Design review of the part built by this model. Coordinates are the model's own, in mm. A direction names the side the tool comes from. Give positions to 0.01 mm unless a question says otherwise; leave off trailing zeros. Loops run counter-clockwise (first coordinate to the right, second up) from the corner with the lowest first, then second, coordinate; pieces in that order, holes last. Notation, with made-up numbers: M 25,-34 L 83,-34 A19 cw 83,-18 Z; hole C 34,-33.75 d4. An arc over 180 degrees is marked long. Use a Markdown table: item, result. Add a question column.
(1) Insertion check: pin 1 Ø2 at (y, z) = (4, 2) entering from +X; pin 2 Ø0.6 at (x, z) = (1, 2.5) entering from -Y; pin 3 Ø2 at (y, z) = (3, 4.5) entering from -X. Each pin has a flat end and moves straight along its axis. Give the tip position at first contact, or say it passes through.
(2) Draft analysis for pull direction X (two halves, no side actions). For faces 3 (the face through (3, 56, 3)), 4 (the face through (1.5, 3, 4)), 5 (the face through (2.766, 33.785, 3.549)), state which applies: pulls with the +X half, pulls with the -X half, needs draft (parallel to the pull), parting line crosses it, or undercut.
(3) For probe 1 along Y at (x, z) = (3, 5); probe 2 along Y at (x, z) = (2.35, 3.5); probe 3 along Y at (x, z) = (5.05, 5.5), list the stretches that pass through material, from the lowest coordinate up.
(4) Add section C-C, the plane x = 3. Give the boundary of the cut face in (y, z).
(5) Add section A-A, the plane y = 32. Give the boundary of the cut face in (x, z).
(6) Add section B-B, the plane z = 0.5. Give the boundary of the cut face in (x, y), then the cut area to 3 significant figures.
(7) For faces 1 (the face through (4.5, 3, 4)), 2 (the face through (6, 31, 3)), list the 3-axis set-ups (+Z, -Z, +X, -X, +Y, -Y) from which the entire face can be reached by the end or side of a thin tool; tool diameter is ignored.
```python
from build123d import *

# Parameters (mm, degrees)
F0_W     = 6
F0_H     = 56
F1_DEPTH = 7
F2_R     = 1.8
F3_DEPTH = 7.001
F4_W     = 1.5
F4_H     = 7
F5_DEPTH = 7.001
F6_R     = 0.5


with BuildPart() as f1:
    # F0 (on Top) → F1 (new body)
    with BuildSketch(Plane.XY):
        with Locations((3, 28)):
            Rectangle(F0_W, F0_H)
    extrude(amount=F1_DEPTH)

    # F2 (on face) → F3 (cut, through all)
    with BuildSketch(Plane.XY.offset(7)):
        with Locations((3, 52)):
            Circle(F2_R)
        with Locations((3, 32)):
            Circle(F2_R)
    extrude(amount=-F3_DEPTH, mode=Mode.SUBTRACT)

    # F4 (on face) → F5 (cut, through all)
    with BuildSketch(Plane.XY.offset(7)):
        with Locations((0.75, 3.5)):
            Rectangle(F4_W, F4_H)
        with Locations((5.25, 3.5)):
            Rectangle(F4_W, F4_H)
    extrude(amount=-F5_DEPTH, mode=Mode.SUBTRACT)

    # F6
    f6_edges = [f1.edges().sort_by_distance(p)[0] for p in [
        (6, 7, 3.5),
        (0, 7, 3.5),
        (4.5, 7, 3.5),
        (1.5, 7, 3.5),
    ]]
    fillet(f6_edges, radius=F6_R)


solid = f1.part
```
Established:
| question | item | result |
|---|---|---|
| 1 | pin 1 | x = 4.5 |
| 1 | pin 2 | y = 6.9 |
| 1 | pin 3 | x = 1.5 |
| 2 | face 3 | needs draft |
| 2 | face 4 | pulls with the -X half |
| 2 | face 5 | undercut |
| 3 | probe 1 | 0 to 30.2, 33.8 to 50.2, 53.8 to 56 |
| 3 | probe 2 | 0 to 30.32, 33.68 to 50.32, 53.68 to 56 |
| 3 | probe 3 | 7 to 56 |
| 4 | outline | M 0,0 L 30.2,0 L 30.2,7 L 0,7 Z; M 33.8,0 L 50.2,0 L 50.2,7 L 33.8,7 Z; M 53.8,0 L 56,0 L 56,7 L 53.8,7 Z |
| 5 | outline | M 0,0 L 1.2,0 L 1.2,7 L 0,7 Z; M 4.8,0 L 6,0 L 6,7 L 4.8,7 Z |
| 6 | outline | M 0,7.5 A0.5 ccw 0.5,7 L 1,7 A0.5 cw 1.5,6.5 L 1.5,0 L 4.5,0 L 4.5,6.5 A0.5 cw 5,7 L 5.5,7 A0.5 ccw 6,7.5 L 6,56 L 0,56 Z; hole C 3,32 d3.6; hole C 3,52 d3.6 |
| 6 | area | 295 mm^2 |
| 7 | face 1 | +Z, -Z, +X, -Y |
| 7 | face 2 | +Z, -Z, +X, +Y, -Y |
